Geometry: final body of the model. Coordinates: model frame, mm. A direction names the side the tool comes from. Give positions to 0.01 mm unless a question says otherwise; leave off trailing zeros. Write each loop counter-clockwise with the first axis right and the second up, starting at its lowest first coordinate (ties: lowest second). Pieces come first, ordered by that corner, then holes.
from build123d import *

# Parameters (mm, degrees)
BOSS_EXTRUDE1_DEPTH   = 38.1
SKETCH2_W             = 21.59
SKETCH2_H             = 254
CUT_EXTRUDE1_DEPTH    = 27.94
CUT_EXTRUDE8_DEPTH    = 86.725
SKETCH12_W            = 19.558
SKETCH12_H            = 12.7
CUT_EXTRUDE9_DEPTH    = 131.908603613
SKETCH13_R            = 2.413
CUT_EXTRUDE10_DEPTH   = 71.997998035
F_8_CLEARANCE_HOLE1_D = 4.4958
FILLET2_R             = 5.08


with BuildPart() as part:
    # Sketch1 → Boss-Extrude1 (new body)
    with BuildSketch(Plane(origin=(0, 0, 0), x_dir=(1, 0, 0), z_dir=(0, 1, 0))):
        Polygon((-19.05, 60.325), (-19.05, 66.675), (19.029461499, 66.675), (19.05, 60.325), (19.05, -60.325), (-19.05, -60.325), align=None)
    extrude(amount=BOSS_EXTRUDE1_DEPTH)

    # Sketch2 → Cut-Extrude1 (cut)
    with BuildSketch(Plane(origin=(0, 38.1, 0), x_dir=(1, 0, 0), z_dir=(0, 1, 0))):
        with Locations((0, -31.75)):
            Rectangle(SKETCH2_W, SKETCH2_H)
    extrude(amount=-CUT_EXTRUDE1_DEPTH, mode=Mode.SUBTRACT)

    # Sketch11 → Cut-Extrude8 (cut, through all)
    with BuildSketch(Plane.ZY.offset(19.05)):
        Polygon((60.325, 25.4), (35.000755529, 25.4), (21.802528375, 25.4), (-28.499244471, 25.4), (-41.697471625, 25.4), (-60.498358048, 25.4), (-66.675, 25.4), (-71.377274135, 25.4), (-71.377274135, 38.1), (-66.675, 38.1), (-60.498358048, 38.1), (60.325, 38.1), align=None)
    extrude(amount=-CUT_EXTRUDE8_DEPTH, mode=Mode.SUBTRACT)

    # Sketch12 → Cut-Extrude9 (cut, through all)
    with BuildSketch(Plane.XY.offset(60.325)):
        Rectangle(SKETCH12_W, SKETCH12_H)
    extrude(amount=-CUT_EXTRUDE9_DEPTH, mode=Mode.SUBTRACT)

    # Sketch13 → Cut-Extrude10 (cut, through all)
    with BuildSketch(Plane(origin=(0, 10.16, 0), x_dir=(1, 0, 0), z_dir=(0, 1, 0))):
        with Locations(Location((0, -53.975, 0), (0, 0, 270))):
            Circle(SKETCH13_R)
        with Locations(Location((0, 47.625, 0), (0, 0, 270))):
            Circle(SKETCH13_R)
        with Locations(Location((0, -3.175, 0), (0, 0, 270))):
            Circle(SKETCH13_R)
    extrude(amount=-CUT_EXTRUDE10_DEPTH, mode=Mode.SUBTRACT)

    # #8 Clearance Hole1 (through all)
    with Locations(Plane(origin=(0, 25.4, 0), x_dir=(1, 0, 0), z_dir=(0, 1, 0))):
        with Locations((-14.9225, -36.530628157), (-14.9225, -7.955628157), (14.9225, -7.955628157), (14.9225, -36.530628157)):
            Hole(F_8_CLEARANCE_HOLE1_D / 2)

    # Fillet2
    fillet2_edges = [part.edges().sort_by_distance(p)[0] for p in [
        (14.4145, 0, 60.325),
        (14.9225, 25.4, 60.325),
        (-14.9225, 25.4, 60.325),
        (-14.4145, 0, 60.325),
    ]]
    fillet(fillet2_edges, radius=FILLET2_R)


solid = part.part
Q1. Section C-C on z = -52.5. Output: boundary loops of the cut face in (x, y) (3 decimals), plus the area to 3 significant figures.
Filled sheet:
outline: (-19.05, 0) - (-9.779, 0) - (-9.779, 6.35) - (9.779, 6.35) - (9.779, 0) - (19.05, 0) - (19.05, 25.4) - (10.795, 25.4) - (10.795, 10.16) - (-10.795, 10.16) - (-10.795, 25.4) - (-19.05, 25.4) - close
area: 515 mm2
Q2. Access query for faces 1 (the flat face through (9.779, 3, -2)), 2 (the flat face through (0, 10.16, -4)), 3 (the flat face through (0, 9, 60.325)). Directions: +Z, -Z, +X, -X, +Y, -Y. A direction counts if a zero-diameter tool reaches every point of the face in a straight line with its end or side. Return the directions, or none.
Filled sheet:
face 1: +Z, -Z, -Y
face 2: +Z, -Z, +Y
face 3: +Z, +X, -X, +Y, -Y
Q3. Section A-A on y = 17.25. Count the separate pieces of the cut face and the enclosed holes in it, plus the area to 3 significant figures.
Filled sheet:
separate pieces: 2
enclosed holes: 4
area: 2,030 mm2
Q4. Section D-D on x = 14.5. Output: boundary loops of the cut face in (y, z) (3 decimals), plus the area to 3 significant figures.
Filled sheet:
outline: (0, -66.675) - (25.4, -66.675) - (25.4, 5.748) - (0, 5.748) - close; (0, 10.163) - (25.4, 10.163) - (25.4, 34.323) - (0, 34.323) - close; (0, 38.738) - (25.4, 38.738) - (25.4, 55.245) arc R5.08 ccw to (20.32, 60.325) - (5.08, 60.325) arc R5.08 ccw to (0, 55.245) - close
area: 2,990 mm2
Q5. Pull-direction query (X, two-part tool) for faces 4 (the flat face through (-9.779, 3, -2)), 5 (the cylindrical face through (-14.86, 23.87, 58.88)), 6 (the cylindrical face through (-16.131, 12.522, 34.635)); classes: released by +X, released by -X, zero draft, split by the parting line, or undercut.
Filled sheet:
face 4: undercut
face 5: zero draft
face 6: undercut
Q6. Pin query (flat end, axial travel): P1, Ø2.5, axis at x = -14.92, z = 36.53, coming from the +Y side; P2, Ø1.5, axis at x = -4, z = -13, coming from the -Y side; P3, Ø6, axis at x = -5, z = 7.5, coming from the +Y side. Return the tip coordinate at first contact, or that it passes through.
Filled sheet:
P1: passes through
P2: stops at y = 6.35
P3: stops at y = 10.16
Q7. Ray query, line 1 along X through (y, z) = (5.5, -60.5); line 2 along X through (y, z) = (19, -51.5) (3 decimals); line 3 along Z through (x, y) = (15.5, 18) (3 decimals). Return the intervals inside material, ascending.
Filled sheet:
line 1: x = -19.05 to -9.78, 9.78 to 19.05
line 2: x = -19.05 to -10.795, 10.795 to 19.05
line 3: z = -66.675 to 5.783, 10.128 to 34.358, 38.703 to 60.325
Q8. Section B-B on x = 0. Output: boundary loops of the cut face in (y, z) (3 decimals).
Filled sheet:
outline: (6.35, -66.675) - (10.16, -66.675) - (10.16, -50.038) - (6.35, -50.038) - close; (6.35, -45.212) - (10.16, -45.212) - (10.16, 0.762) - (6.35, 0.762) - close; (6.35, 5.588) - (10.16, 5.588) - (10.16, 51.562) - (6.35, 51.562) - close; (6.35, 56.388) - (10.16, 56.388) - (10.16, 60.325) - (6.35, 60.325) - close
